from build123d import *

# Parameters (mm, degrees)
FILLET1_R          = 5
CUT_EXTRUDE1_START = -3
CUT_EXTRUDE1_DEPTH = 3.4
SKETCH3_R          = 2.1
CUT_EXTRUDE2_DEPTH = 12
CHAMFER1_SIZE      = 5


# Read off the part's stored shape, not the designer's step: Revolve-Thin2
with BuildPart() as part:
    # Revolve-Thin2 outline → Revolve-Thin2 (revolve)
    with BuildSketch(Plane.XY):
        Polygon((0, 60), (0, 0), (15, 0), (15, 5), (10, 5), (10, 55), (15, 55), (15, 60), align=None)
    revolve(axis=Axis((0, 0, 0), (0, 1, 0)))

    # Fillet1
    fillet1_edges = [part.edges().sort_by_distance(p)[0] for p in [
        (-10, 5, 0),
    ]]
    fillet(fillet1_edges, radius=FILLET1_R - 0.0001)  # a hair under: the kernel refuses the full size

    # Sketch2 → Cut-Extrude1 (cut)
    with BuildSketch(Plane(origin=(0, 60, 0), x_dir=(1, 0, 0), z_dir=(0, 1, 0)).offset(CUT_EXTRUDE1_START)):
        Polygon((0, 4.099186911), (-3.55, 2.049593456), (-3.55, -2.049593456), (0, -4.099186911), (3.55, -2.049593456), (3.55, 2.049593456), align=None)
    extrude(amount=-CUT_EXTRUDE1_DEPTH, mode=Mode.SUBTRACT)

    # Sketch3 → Cut-Extrude2 (cut)
    with BuildSketch(Plane(origin=(0, 60, 0), x_dir=(1, 0, 0), z_dir=(0, 1, 0))):
        with Locations(Location((0, 0, 0), (0, 0, 270))):
            Circle(SKETCH3_R)
    extrude(amount=-CUT_EXTRUDE2_DEPTH, mode=Mode.SUBTRACT)

    # Chamfer1
    chamfer1_edges = [part.edges().sort_by_distance(p)[0] for p in [
        (-15, 55, 0),
    ]]
    chamfer(chamfer1_edges, length=CHAMFER1_SIZE - 0.0001)  # a hair under: the kernel refuses the full size


solid = part.part
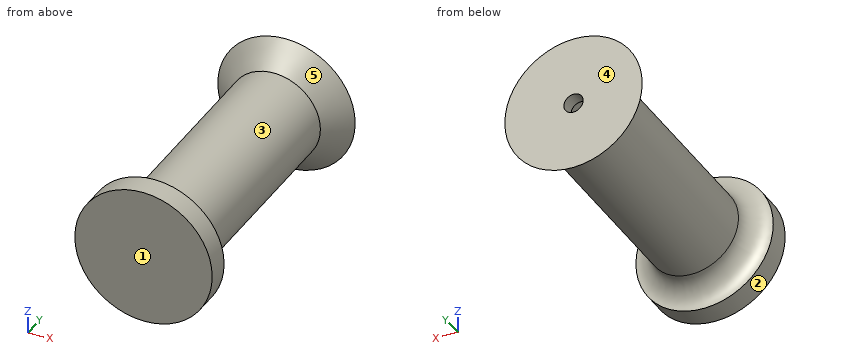
Check sheet for the modelled part. Datum: model origin and axes. Units: mm. Face numbers are marked on the shaded views. A direction names the side the tool comes from. Round coordinates to 2 decimals unless told otherwise and drop trailing zeros. Loops run counter-clockwise (first coordinate to the right, second up) from the corner with the lowest first, then second, coordinate; pieces in that order, holes last. Notation, with made-up numbers: (30, -19.75) -> (78, -19.75) arc R22 cw to (78, 10.25) -> close; hole circle Ø3 at (81.5, -18). An arc over 180 degrees is marked (long way). Put each result on its own line as item: value. Start each with the question number.
1. Section check D-D (y = 6.5). Enter the section's corners in (x, z).
2. Scan lines: probe 1 along X at (y, z) = (51.7, 0); probe 2 along Y at (x, z) = (12.5, 5.75); probe 3 along X at (y, z) = (58.7, 0). Record each from-to range of solid material in increasing order.
3. Draft check along Y on the marked faces 1, 2 and 3. Enter one of: +Y half, -Y half, draft (parallel to the pull), parting line (faces both ways), or undercut.
4. Access from +Z, -Z, +X, -X, +Y, -Y to the whole of each face (thin tool, end or side, straight path). Record for the marked faces 4 and 5.
5. Section check C-C (y = 38). Enter the section's corners in (x, z).
6. Gauge pin test, flat ends, axial feed: pin 1 (16 mm diameter, centred on x = 0, z = 3.5, fed in from -Y); pin 2 (4 mm diameter, centred on y = 12, z = -8.5, fed in from -X); pin 3 (4 mm diameter, centred on x = 3, y = 31, fed in from -Z); pin 4 (3.5 mm diameter, centred on y = 56, z = -1, fed in from +X). Record the tip position at first contact, or that the pin passes through.
7. Section check A-A (y = 49.5). Enter the section's corners in (x, z).
Findings:
1. outline: circle Ø22.86 at (0, 0)
2. probe 1: x = -10 to -2.1, 2.1 to 10
2. probe 2: y = 0 to 5.16, 58.76 to 60
2. probe 3: x = -13.7 to -2.1, 2.1 to 13.7
3. face 1: -Y half
3. face 2: draft
3. face 3: undercut
4. face 4: +Z, -Z, +X, -X, +Y
4. face 5: none
5. outline: circle Ø20 at (0, 0)
6. pin 1: stops at y = 0
6. pin 2: stops at x = -7.6
6. pin 3: stops at z = -9.95
6. pin 4: stops at x = 12.72
7. outline: circle Ø20 at (0, 0); hole circle Ø4.2 at (0, 0)
